The listing builds one solid part. Answer for the finished solid, in the listing's coordinates (mm). A direction names the side the tool comes from. Give positions to 0.01 mm unless a question says otherwise; leave off trailing zeros. Write each loop counter-clockwise with the first axis right and the second up, starting at its lowest first coordinate (ties: lowest second). Pieces come first, ordered by that corner, then holes. Notation, with made-up numbers: (14, 83) -> (70, 83) arc R19 ccw to (70, 96) -> close; hole circle Ø9 at (56, 14.25). An arc over 180 degrees is marked (long way). Put each result on its own line as item: value. Start each with the question number.
1) Flat-ended cylindrical pins translate along their axes: pin 1 Ø4.5 at (x, z) = (-17.29, 49.7) entering from -Y; pin 2 Ø2 at (y, z) = (-2, 20.5) entering from +X. Find the tip coordinate at first contact, or state that the pin passes through.
2) For faces 1 (the flat face through (-30, 0, 24)), 2 (the flat face through (-32.067, -3.219, 26.647)), determine the directions among +Z, -Z, +X, -X, +Y, -Y from which every point of the face is accessible in a straight line to the end or side of a thin tool.
3) Find the intervals of material crossed by line 1 along Z through (x, y) = (-49, -6); line 2 along X through (y, z) = (-2, 51.5); line 3 along X through (y, z) = (-2.75, 47.5), in increasing order. Write a range as from..to.
4) A cutting plane is placed at A-A (y = -5.5). Write down the section's boundary in (x, z), then the cut area to 3 significant figures.
5) A cutting plane is placed at D-D (z = 50.5). Write down the section's boundary in (x, y), then the cut area to 3 significant figures.
6) A cutting plane is placed at C-C (z = 25.5). Write down the section's boundary in (x, y), then the cut area to 3 significant figures.
7) A cutting plane is placed at B-B (x = -33.5). Write down the section's boundary in (y, z).
from build123d import *

# Parameters (mm, degrees)
F1_DEPTH = 6.35
F3_DEPTH = 25.4
F4_R     = 5.08
F5_R     = 5.08
F7_D     = 4.9276


with BuildPart() as f1:
    # F0 (on Front) → F1 (new body)
    with BuildSketch(Plane.XZ):
        Polygon((-8.49073, 54.782512), (-75.920123, 54.782512), (-75.920123, 3.982512), (-37.820123, 3.982512), align=None)
    extrude(amount=F1_DEPTH)

    # F2 (on face) → F3 (cut)
    with BuildSketch(Plane.XZ.offset(6.35)):
        Polygon((-41.486298, 10.332512), (-19.489252, 48.432512), (-69.570123, 48.432512), (-69.570123, 10.332512), align=None)
    extrude(amount=-F3_DEPTH, mode=Mode.SUBTRACT)

    # F4
    f4_edges = [f1.edges().sort_by_distance(p)[0] for p in [
        (-8.49073, -3.175, 54.782512),
        (-75.920123, -3.175, 54.782512),
        (-37.820123, -3.175, 3.982512),
        (-75.920123, -3.175, 3.982512),
    ]]
    fillet(f4_edges, radius=F4_R)

    # F5
    f5_edges = [f1.edges().sort_by_distance(p)[0] for p in [
        (-41.486298, -3.175, 10.332512),
        (-69.570123, -3.175, 10.332512),
        (-69.570123, -3.175, 48.432512),
        (-19.489252, -3.175, 48.432512),
    ]]
    fillet(f5_edges, radius=F5_R)

    # F7 (through all)
    with Locations(Plane.XZ.offset(6.35)):
        with Locations((-70.840123, 49.702512), (-70.840123, 9.062512), (-17.289548, 49.702512)):
            Hole(F7_D / 2)


solid = f1.part
Reply:
1. pin 1: passes through
1. pin 2: stops at x = -27.71
2. face 1: +Z, -Z, +X, -X, +Y
2. face 2: +Y, -Y
3. line 1: z = 3.98..10.33, 48.43..54.78
3. line 2: x = -75.59..-72.53, -69.16..-18.97, -15.6..-12.54
3. line 3: x = -75.92..-71.94, -69.74..-67.42, -25.35..-18.39, -16.19..-12.71
4. outline: (-75.92, 9.06) arc R5.08 ccw to (-70.84, 3.98) -> (-40.75, 3.98) arc R5.08 ccw to (-36.35, 6.52) -> (-12.89, 47.16) arc R5.08 ccw to (-17.29, 54.78) -> (-70.84, 54.78) arc R5.08 ccw to (-75.92, 49.7) -> close; hole circle Ø4.93 at (-70.84, 9.06); hole circle Ø4.93 at (-70.84, 49.7); hole (-69.57, 15.41) arc R5.08 ccw to (-64.49, 10.33) -> (-44.42, 10.33) arc R5.08 ccw to (-40.02, 12.87) -> (-23.89, 40.81) arc R5.08 ccw to (-28.29, 48.43) -> (-64.49, 48.43) arc R5.08 ccw to (-69.57, 43.35) -> close; hole circle Ø4.93 at (-17.29, 49.7)
4. area: 1,130 mm2
5. outline: (-75.86, -6.35) -> (-73.17, -6.35) -> (-73.17, 0) -> (-75.86, 0) -> close; (-68.51, -6.35) -> (-19.62, -6.35) -> (-19.62, 0) -> (-68.51, 0) -> close; (-14.96, -6.35) -> (-12.27, -6.35) -> (-12.27, 0) -> (-14.96, 0) -> close
5. area: 345 mm2
6. outline: (-75.92, -6.35) -> (-69.57, -6.35) -> (-69.57, 0) -> (-75.92, 0) -> close; (-32.73, -6.35) -> (-25.4, -6.35) -> (-25.4, 0) -> (-32.73, 0) -> close
6. area: 86.9 mm2
7. outline: (-6.35, 11.47) -> (0, 11.47) -> (0, 24.17) -> (-6.35, 24.17) -> close; (-6.35, 48.43) -> (0, 48.43) -> (0, 54.78) -> (-6.35, 54.78) -> close
